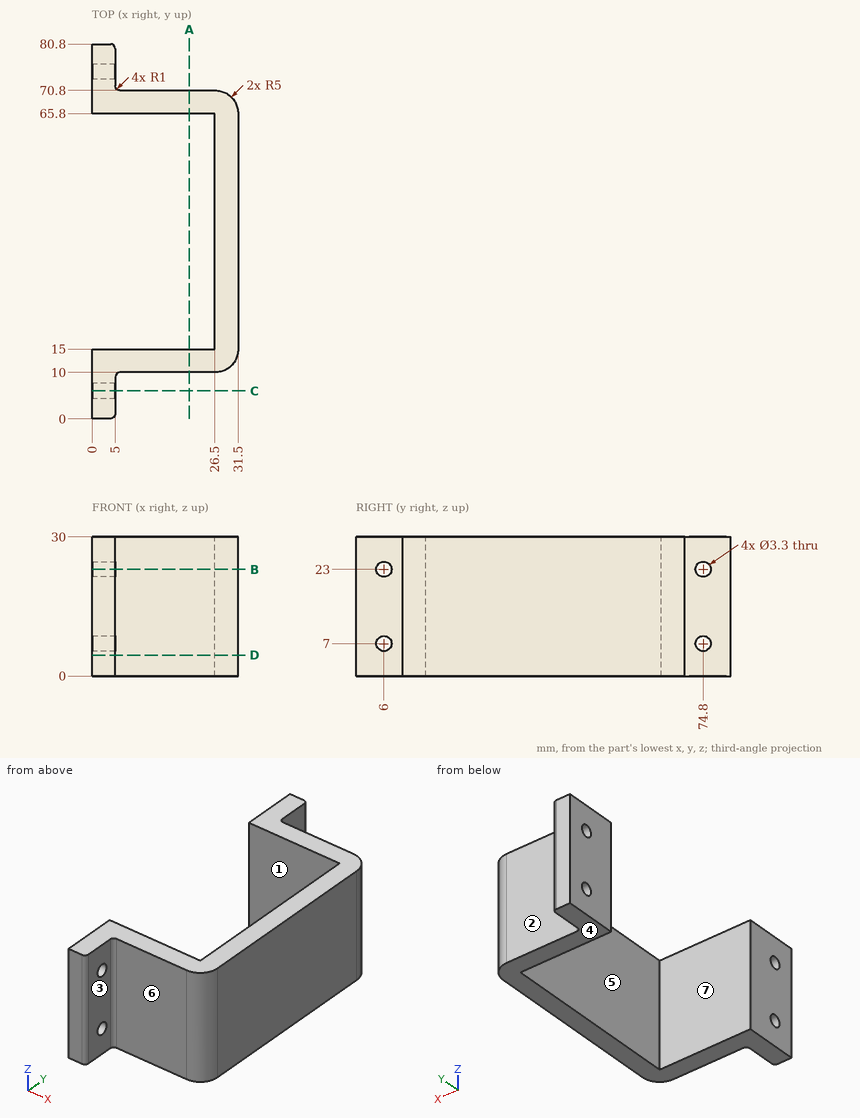
Study the drawing (mm; zero at the part's minimum x, y, z) and answer. A direction names the side the tool comes from. Give positions to 0.01 mm unless a question says otherwise; leave off trailing zeros. Order: outer loops, then holes, each group sorted by start corner. A loop starts at its lowest first (then second) coordinate and runs counter-clockwise, first axis right, second up.
1) Find section D-D on z = 4.5. Write down the section's boundary in (x, y), then the cut area to 3 significant figures.
Reported:
outline: (0, 0) - (4, 0) arc R1 ccw to (5, 1) - (5, 9) arc R1 cw to (6, 10) - (26.5, 10) arc R5 ccw to (31.5, 15) - (31.5, 65.8) arc R5 ccw to (26.5, 70.8) - (6, 70.8) arc R1 cw to (5, 71.8) - (5, 79.8) arc R1 ccw to (4, 80.8) - (0, 80.8) - (0, 65.8) - (26.5, 65.8) - (26.5, 15) - (0, 15) - close
area: 658 mm2
2) Determine the mould class of the marked faces 4, 5, 6 and 7 for opening direction Y: pulls with the +Y half, pulls with the -Y half, needs draft (parallel to the pull), parting line crosses it, or undercut.
Reported:
face 4: needs draft
face 5: undercut
face 6: pulls with the -Y half
face 7: undercut
3) Find section C-C on y = 6. Write down the section's boundary in (x, z), then the cut area to 3 significant figures.
Reported:
outline: (0, 0) - (5, 0) - (5, 5.35) - (0, 5.35) - close; (0, 8.65) - (5, 8.65) - (5, 21.35) - (0, 21.35) - close; (0, 24.65) - (5, 24.65) - (5, 30) - (0, 30) - close
area: 117 mm2
4) Given P1, Ø2.5, axis at y = 74.8, z = 7, coming from the +X side; P2, Ø9, axis at y = 35.5, z = 16, coming from the -X side; P3, Ø1.5, axis at x = 20, z = 5, coming from the +Y side; P4, Ø4, axis at y = 77, z = 8.5, coming from the +X side, each flat-ended and moving along its own axis, determine where each tip first touches the part or whether it passes through.
Reported:
P1: passes through
P2: stops at x = 26.5
P3: stops at y = 70.8
P4: stops at x = 5
5) Find section B-B on z = 23. Write down the section's boundary in (x, y).
Reported:
outline: (0, 0) - (4, 0) arc R1 ccw to (5, 1) - (5, 4.35) - (0, 4.35) - close; (0, 7.65) - (5, 7.65) - (5, 9) arc R1 cw to (6, 10) - (26.5, 10) arc R5 ccw to (31.5, 15) - (31.5, 65.8) arc R5 ccw to (26.5, 70.8) - (6, 70.8) arc R1 cw to (5, 71.8) - (5, 73.15) - (0, 73.15) - (0, 65.8) - (26.5, 65.8) - (26.5, 15) - (0, 15) - close; (0, 76.45) - (5, 76.45) - (5, 79.8) arc R1 ccw to (4, 80.8) - (0, 80.8) - close
6) For the marked faces 1, 2 and 3, determine the directions among +Z, -Z, +X, -X, +Y, -Y from which every point of the face is accessible in a straight line to the end or side of a thin tool.
Reported:
face 1: +Z, -Z, -X
face 2: +Z, -Z, +X, +Y
face 3: +Z, -Z, +X, -Y
7) Consider line 1 along Z through (x, y) = (4, 74.8); line 2 along Y through (x, z) = (3.2, 23); line 3 along Y through (x, z) = (3.5, 14.5). Determine where each line is inside the solid, lowest interval first.
Reported:
line 1: z = 0 to 5.35, 8.65 to 21.35, 24.65 to 30
line 2: y = 0 to 4.35, 7.65 to 15, 65.8 to 73.15, 76.45 to 80.8
line 3: y = 0 to 15, 65.8 to 80.8
8) Find section A-A on x = 21. Write down the section's boundary in (y, z), then the cut area to 3 significant figures.
Reported:
outline: (10, 0) - (15, 0) - (15, 30) - (10, 30) - close; (65.8, 0) - (70.8, 0) - (70.8, 30) - (65.8, 30) - close
area: 300 mm2
